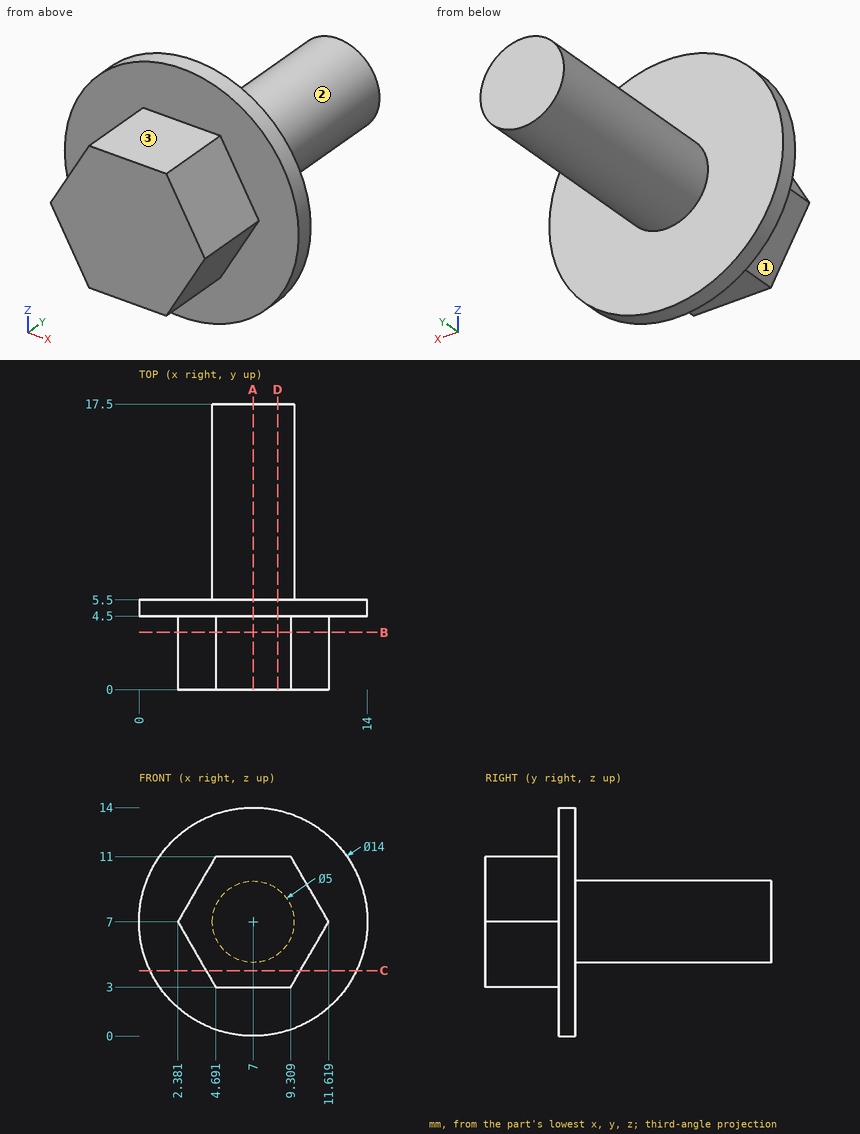
Design review of the part shown in the three views and the two pictorial views. Dimensions are in mm from the part's minimum x, y and z. A direction names the side the tool comes from. Round coordinates to 2 decimals unless told otherwise and drop trailing zeros. Loops run counter-clockwise (first coordinate to the right, second up) from the corner with the lowest first, then second, coordinate; pieces in that order, holes last. Notation, with made-up numbers: (50.5, 6) - (90.5, 6) arc R19 cw to (90.5, 40) - close; hole circle Ø3 at (43, 49). An arc over 180 degrees is marked (long way). Use one line per item in the form item = value.
1) We need section B-B on y = 3.5. Write out the cut boundary in (x, z), then the cut area to 3 significant figures.
Solutions:
outline = (2.38, 7) - (4.69, 3) - (9.31, 3) - (11.62, 7) - (9.31, 11) - (4.69, 11) - close
area = 55.4 mm2
2) We need section A-A on x = 7. Write out the cut boundary in (y, z).
Solutions:
outline = (0, 3) - (4.5, 3) - (4.5, 0) - (5.5, 0) - (5.5, 4.5) - (17.5, 4.5) - (17.5, 9.5) - (5.5, 9.5) - (5.5, 14) - (4.5, 14) - (4.5, 11) - (0, 11) - close
3) Clearance check with flat-ended pins moving along their axes: P1, Ø3, axis at y = 14.5, z = 8, coming from the +X side; P2, Ø6, axis at y = 2.5, z = 9.5, coming from the +X side (1 decimal); P3, Ø8, axis at x = 11, y = 11, coming from the +Z side. State where each tip first meets the part, or that it passes through.
Solutions:
P1 = 9.5
P2 = 14
P3 = 9.5
4) Tool access review of the marked faces 1, 2 and 3: name each direction out of +Z, -Z, +X, -X, +Y, -Y from which nothing blocks a thin tool from reaching the whole face with its end or side.
Solutions:
face_1 = -Z, -X, -Y
face_2 = +Y
face_3 = +Z, +X, -X, -Y
5) Wall thickness on probe 1 along Y at (x, z) = (2, 7); probe 2 along Y at (x, z) = (9, 10.25); probe 3 along Z at (x, y) = (6.5, 12): over which ranges is each line inside the solid? List them lowest first.
Solutions:
probe_1 = 4.5 to 5.5
probe_2 = 0 to 5.5
probe_3 = 4.55 to 9.45
6) We need section C-C on z = 4. Write out the cut boundary in (x, y) (1 decimal).
Solutions:
outline = (0.7, 4.5) - (4.1, 4.5) - (4.1, 0) - (9.9, 0) - (9.9, 4.5) - (13.3, 4.5) - (13.3, 5.5) - (0.7, 5.5) - close
7) We need section D-D on x = 8.5. Write out the cut boundary in (y, z).
Solutions:
outline = (0, 3) - (4.5, 3) - (4.5, 0.16) - (5.5, 0.16) - (5.5, 5) - (17.5, 5) - (17.5, 9) - (5.5, 9) - (5.5, 13.84) - (4.5, 13.84) - (4.5, 11) - (0, 11) - close
